from build123d import *

# Parameters (mm, degrees)
SKETCH1_W                = 60
SKETCH1_H                = 5
BOSS_EXTRUDE1_DEPTH      = 391
SKETCH3_W                = 250
SKETCH3_H                = 5
BOSS_EXTRUDE2_DEPTH      = 95
SKETCH4_R                = 2.5
CUT_EXTRUDE1_DEPTH       = 95
SKETCH5_W                = 50
SKETCH5_H                = 141
BOSS_EXTRUDE3_DEPTH      = 5
SKETCH6_W                = 5
SKETCH6_H                = 50
BOSS_EXTRUDE4_DEPTH      = 80
SKETCH7_R                = 5
CUT_EXTRUDE2_DEPTH       = 40
CUT_EXTRUDE3_DEPTH       = 10
SKETCH11_W               = 40
SKETCH11_H               = 5
BOSS_EXTRUDE5_DEPTH      = 10
SKETCH12_W               = 30
SKETCH12_H               = 5
SKETCH12_W_2             = 17.5
BOSS_EXTRUDE6_DEPTH      = 10
SKETCH14_W               = 9
SKETCH14_H               = 5
CUT_EXTRUDE4_DEPTH       = 10
SKETCH15_W               = 5
SKETCH15_H               = 90
SKETCH15_H_2             = 50
BOSS_EXTRUDE7_DEPTH      = 15
BOSS_EXTRUDE7_DEPTH_BACK = 20
SKETCH16_W               = 50
SKETCH16_H               = 5
BOSS_EXTRUDE8_DEPTH      = 3
SKETCH18_W               = 90
SKETCH18_H               = 5
BOSS_EXTRUDE9_DEPTH      = 3
SKETCH19_R               = 2.5
CUT_EXTRUDE5_DEPTH       = 28
SKETCH20_W               = 50
SKETCH20_H               = 4.954602057
BOSS_EXTRUDE10_DEPTH     = 70
SKETCH21_R               = 5
CUT_EXTRUDE6_DEPTH       = 70
SKETCH22_R               = 2.5
CUT_EXTRUDE7_DEPTH       = 10
SKETCH23_R               = 5
CUT_EXTRUDE8_DEPTH       = 10


with BuildPart() as part:
    # Sketch1 → Boss-Extrude1 (new body)
    with BuildSketch(Plane.XY):
        Rectangle(SKETCH1_W, SKETCH1_H)
    extrude(amount=BOSS_EXTRUDE1_DEPTH)

    # Sketch3 → Boss-Extrude2 (add)
    with BuildSketch(Plane.ZY.offset(30)):
        with Locations((266, 0)):
            Rectangle(SKETCH3_W, SKETCH3_H)
    extrude(amount=BOSS_EXTRUDE2_DEPTH)

    # Sketch4 → Cut-Extrude1 (cut)
    with BuildSketch(Plane.XZ.offset(2.5)):
        with Locations((-115.67, 250.12)):
            Circle(SKETCH4_R)
        with Locations((-25.67, 250.12)):
            Circle(SKETCH4_R)
        with Locations((-25.67, 270.12)):
            Circle(SKETCH4_R)
        with Locations((-25.67, 290.12)):
            Circle(SKETCH4_R)
        with Locations((-25.67, 310.12)):
            Circle(SKETCH4_R)
        with Locations((-25.67, 330.12)):
            Circle(SKETCH4_R)
        with Locations((-25.67, 350.12)):
            Circle(SKETCH4_R)
        with Locations((-115.67, 270.12)):
            Circle(SKETCH4_R)
        with Locations((-115.67, 290.12)):
            Circle(SKETCH4_R)
        with Locations((-115.67, 310.12)):
            Circle(SKETCH4_R)
        with Locations((-115.67, 330.12)):
            Circle(SKETCH4_R)
        with Locations((-115.67, 350.12)):
            Circle(SKETCH4_R)
        with BuildLine():
            Line((-33.84, 391), (-33.84, 250.12))
            ThreePointArc((-33.84, 250.12), (-70.67, 213.29), (-107.5, 250.12))
            Line((-107.5, 250.12), (-107.5, 391))
            ThreePointArc((-107.5, 391), (-70.67, 427.83), (-33.84, 391))
        make_face()
    extrude(amount=-CUT_EXTRUDE1_DEPTH, mode=Mode.SUBTRACT)

    # Sketch5 → Boss-Extrude3 (add)
    with BuildSketch(Plane.XZ.offset(2.5)):
        with Locations((-65, 70.5)):
            Rectangle(SKETCH5_W, SKETCH5_H)
    extrude(amount=-BOSS_EXTRUDE3_DEPTH)

    # Sketch6 → Boss-Extrude4 (add)
    with BuildSketch(Plane.XZ.offset(2.5)):
        with Locations((-42.5, 25)):
            Rectangle(SKETCH6_W, SKETCH6_H)
    boss_extrude4 = extrude(amount=BOSS_EXTRUDE4_DEPTH)

    # Sketch7 → Cut-Extrude2 (cut)
    with BuildSketch(Plane.ZY.offset(45)):
        with Locations((25, -42.5)):
            Circle(SKETCH7_R)
    cut_extrude2 = extrude(amount=-CUT_EXTRUDE2_DEPTH, mode=Mode.SUBTRACT)

    # Sketch8 → Cut-Extrude3 (cut)
    with BuildSketch(Plane(origin=(0, -2.5, 0), x_dir=(-1, 0, 0), z_dir=(0, -1, 0))):
        Polygon((30, -141), (0, -141), (-13.214015024, -141), (-13.214015024, 0), (0, 0), (30, 0), align=None)
    extrude(amount=-CUT_EXTRUDE3_DEPTH, mode=Mode.SUBTRACT)

    # Sketch11 → Boss-Extrude5 (add)
    with BuildSketch(Plane(origin=(30, 0, 0), x_dir=(0, 0, -1), z_dir=(1, 0, 0))):
        with Locations((-20, 0)):
            Rectangle(SKETCH11_W, SKETCH11_H)
        with Locations((-271, 0)):
            Rectangle(SKETCH11_W, SKETCH11_H)
    extrude(amount=BOSS_EXTRUDE5_DEPTH)

    # Sketch12 → Boss-Extrude6 (add)
    with BuildSketch(Plane.XY.offset(391)):
        with Locations((15, 0)):
            Rectangle(SKETCH12_W, SKETCH12_H)
        with Locations((-116.25, 0)):
            Rectangle(SKETCH12_W_2, SKETCH12_H)
    extrude(amount=BOSS_EXTRUDE6_DEPTH)

    # Mirror1: Boss-Extrude4, Cut-Extrude2 across plane
    add(boss_extrude4.mirror(Plane.ZX))
    add(cut_extrude2.mirror(Plane.ZX), mode=Mode.SUBTRACT)

    # Sketch14 → Cut-Extrude4 (cut)
    with BuildSketch(Plane.XY.offset(401)):
        with Locations((-120.75, 0)):
            Rectangle(SKETCH14_W, SKETCH14_H)
    extrude(amount=-CUT_EXTRUDE4_DEPTH, mode=Mode.SUBTRACT)

    # Sketch15 → Boss-Extrude7 (add, two sides)
    with BuildSketch(Plane.XZ.offset(2.5)) as boss_extrude7_sk:
        with Locations((10.5, 226)):
            Rectangle(SKETCH15_W, SKETCH15_H)
        with Locations((-23, 210)):
            Rectangle(SKETCH15_W, SKETCH15_H_2)
    extrude(amount=BOSS_EXTRUDE7_DEPTH)
    extrude(boss_extrude7_sk.sketch, amount=-BOSS_EXTRUDE7_DEPTH_BACK)

    # Sketch16 → Boss-Extrude8 (add)
    with BuildSketch(Plane(origin=(-20.5, 0, 0), x_dir=(0, 0, -1), z_dir=(1, 0, 0))):
        with Locations((-210, -15)):
            Rectangle(SKETCH16_W, SKETCH16_H)
        with Locations((-210, 15)):
            Rectangle(SKETCH16_W, SKETCH16_H)
    extrude(amount=BOSS_EXTRUDE8_DEPTH)

    # Sketch18 → Boss-Extrude9 (add)
    with BuildSketch(Plane.ZY.offset(-8)):
        with Locations((226, 15)):
            Rectangle(SKETCH18_W, SKETCH18_H)
        with Locations((226, -15)):
            Rectangle(SKETCH18_W, SKETCH18_H)
    extrude(amount=BOSS_EXTRUDE9_DEPTH)

    # Sketch19 → Cut-Extrude5 (cut)
    with BuildSketch(Plane.ZY.offset(45)):
        with Locations((9.5, 58)):
            Circle(SKETCH19_R)
        with Locations((40.5, 58)):
            Circle(SKETCH19_R)
        with Locations((40.5, 27)):
            Circle(SKETCH19_R)
        with Locations((9.5, 27)):
            Circle(SKETCH19_R)
        with Locations((40.5, -27)):
            Circle(SKETCH19_R)
        with Locations((40.5, -58)):
            Circle(SKETCH19_R)
        with Locations((9.5, -58)):
            Circle(SKETCH19_R)
        with Locations((9.5, -27)):
            Circle(SKETCH19_R)
    extrude(amount=-CUT_EXTRUDE5_DEPTH, mode=Mode.SUBTRACT)

    # Sketch20 → Boss-Extrude10 (add)
    with BuildSketch(Plane(origin=(0, 0, 0), x_dir=(-1, 0, 0), z_dir=(0, 0, -1))):
        with Locations((65, -0.022698971)):
            Rectangle(SKETCH20_W, SKETCH20_H)
    extrude(amount=BOSS_EXTRUDE10_DEPTH)

    # Sketch21 → Cut-Extrude6 (cut)
    with BuildSketch(Plane.XZ.offset(2.5)):
        with Locations((-56.5, -38.21)):
            Circle(SKETCH21_R)
    extrude(amount=-CUT_EXTRUDE6_DEPTH, mode=Mode.SUBTRACT)

    # Sketch22 → Cut-Extrude7 (cut)
    with BuildSketch(Plane(origin=(0, 2.5, 0), x_dir=(1, 0, 0), z_dir=(0, 1, 0))):
        with Locations((-77.21, -19)):
            Circle(SKETCH22_R)
    extrude(amount=-CUT_EXTRUDE7_DEPTH, mode=Mode.SUBTRACT)

    # Sketch23 → Cut-Extrude8 (cut)
    with BuildSketch(Plane(origin=(0, 2.5, 0), x_dir=(1, 0, 0), z_dir=(0, 1, 0))):
        with Locations((-107.5, -173.5)):
            Circle(SKETCH23_R)
    extrude(amount=-CUT_EXTRUDE8_DEPTH, mode=Mode.SUBTRACT)


solid = part.part
Geometry check sheet. Reference: the model listing, model coordinates, mm. A direction names the side the tool comes from. Round coordinates to 2 decimals unless told otherwise and drop trailing zeros. Write each loop counter-clockwise with the first axis right and the second up, starting at its lowest first coordinate (ties: lowest second). Pieces come first, ordered by that corner, then holes. Notation, with made-up numbers: (13.5, 19) -> (49.5, 19) arc R36 ccw to (49.5, 58) -> close; hole circle Ø6 at (-25, -7.75). An arc over 180 degrees is marked (long way). One line per item, written item: value. Start each with the question number.
(1) Draft check along Z on faces 5 (the flat face through (10, -10, 181)), 6 (the cylindrical face through (-42.535, 39.121, 21.315)), 7 (the flat face through (-45, -42, 19)). Enter one of: +Z half, -Z half, draft (parallel to the pull), parting line (faces both ways), or undercut.
(2) Go/stop test with flat-tipped pins: pin 1 Ø8 at (x, z) = (-71.5, 75) entering from -Y; pin 2 Ø1.5 at (x, z) = (12, 122.5) entering from -Y; pin 3 Ø6 at (y, z) = (27, 40.5) entering from -X; pin 4 Ø8 at (y, z) = (-58, 9.5) entering from +X. Record where each tip stops, or that it passes through.
(3) Access from +Z, -Z, +X, -X, +Y, -Y to the whole of each face (thin tool, end or side, straight path). Record for faces 1 (the flat face through (13, 10, 225)), 2 (the flat face through (-20.5, 7, 210)), 3 (the flat face through (-25.5, 10, 210)), 4 (the flat face through (10, -10, 271)).
(4) Cross-section at C-C, the plane x = -56.5. Record the cut outline in (y, z) (3 decimals).
(5) Scan lines: line 1 (Y direction, x = -43.55, z = 9.5); line 2 (Y direction, x = -30.5, z = 345.5); line 3 (Z direction, x = -22, y = 5). Record each from-to range of solid material in increasing order. Write a range as [from, to].
(6) Cross-section at A-A, the plane z = 84.5. Record the cut outline in (x, y).
(7) Cross-section at B-B, the plane y = -42.5. Record the cut outline in (x, z), and give its area (3 significant figures).
(8) Cross-section at D-D, the plane z = 241. Record the cut outline in (x, y), and give its area (3 significant figures).
Answer:
1. face 5: -Z half
1. face 6: undercut
1. face 7: draft
2. pin 1: y = -2.5
2. pin 2: through
2. pin 3: x = -45
2. pin 4: x = -40
3. face 1: +Z, -Z, +X, +Y
3. face 2: +Z, -Z
3. face 3: +Z, -Z, -X, +Y
3. face 4: +Z, +X, -X, -Y
4. outline: (-2.5, -70) -> (2.455, -70) -> (2.455, -43.21) -> (-2.5, -43.21) -> close; (-2.5, -33.21) -> (2.455, -33.21) -> (2.455, 0) -> (2.5, 0) -> (2.5, 216.125) -> (-2.5, 216.125) -> close
5. line 1: [-82.5, -60.5], [-55.5, -29.5], [-24.5, 24.5], [29.5, 55.5], [60.5, 82.5]
5. line 2: [-2.5, 2.5]
5. line 3: [185, 235]
6. outline: (-90, -2.5) -> (-40, -2.5) -> (-40, 2.5) -> (-90, 2.5) -> close; (13.21, -2.5) -> (30, -2.5) -> (30, 2.5) -> (13.21, 2.5) -> close
7. outline: (-45, 0) -> (-40, 0) -> (-40, 20) -> (-45, 20) -> close; (-45, 30) -> (-40, 30) -> (-40, 50) -> (-45, 50) -> close
7. area: 200 mm²
8. outline: (-125, -2.5) -> (-106.35, -2.5) -> (-106.35, 2.5) -> (-125, 2.5) -> close; (-34.99, -2.5) -> (8, -2.5) -> (8, -12.5) -> (5, -12.5) -> (5, -17.5) -> (13, -17.5) -> (13, -2.5) -> (30, -2.5) -> (30, 2.5) -> (13, 2.5) -> (13, 17.5) -> (5, 17.5) -> (5, 12.5) -> (8, 12.5) -> (8, 2.5) -> (-34.99, 2.5) -> close
8. area: 598 mm²
